Design review of the part shown in the three views and the two pictorial views. Dimensions are in mm from the part's minimum x, y and z. A direction names the side the tool comes from. Coordinates: 2 decimals unless noted, no trailing zeros. Loops run counter-clockwise (first coordinate to the right, second up) from the corner with the lowest first, then second, coordinate; pieces in that order, holes last. Notation, with made-up numbers: (9, -21) - (63, -21) arc R22 ccw to (63, 8) - close; hole circle Ø1 at (82.5, 82). An arc over 180 degrees is marked (long way). One line per item, written item: value. Start each with the question number.
1. Take a section at A-A, the plane z = 49. State the section outline as (x, y) points (1 decimal), and give its area (3 significant figures).
2. Take a section at B-B, the plane x = 25. State the section outline as (y, z) points (1 decimal), and give its area (3 significant figures).
3. To check wall thickness, follow line 1 (X direction, y = 6.1, z = 5.08) (1 decimal); line 2 (X direction, y = 5, z = 69) (1 decimal); line 3 (Y direction, x = 5.5, z = 97) (1 decimal). State the ranges of each line that lie inside material, in increasing order. Write a range as from..to.
4. For the marked faces 1, 2 and 3, list the 3-axis set-ups (+Z, -Z, +X, -X, +Y, -Y) from which the entire face can be reached by the end or side of a thin tool; tool diameter is ignored.
5. Take a section at C-C, the plane z = 5.08. State the section outline as (x, y) points (1 decimal).
6. Insertion check: pin 1 (6 mm diameter, centred on x = 10.5, z = 27.5, fed in from -Y) (1 decimal); pin 2 (4 mm diameter, centred on x = 14.64, z = 109.22, fed in from -Y) (1 decimal); pin 3 (5 mm diameter, centred on x = 43.5, z = 26, fed in from +Y) (1 decimal). Each pin has a flat end and moves straight along its axis. Give the tip position at first contact, or say it passes through.
7. Take a section at D-D, the plane z = 23.5. State the section outline as (x, y) points (1 decimal).
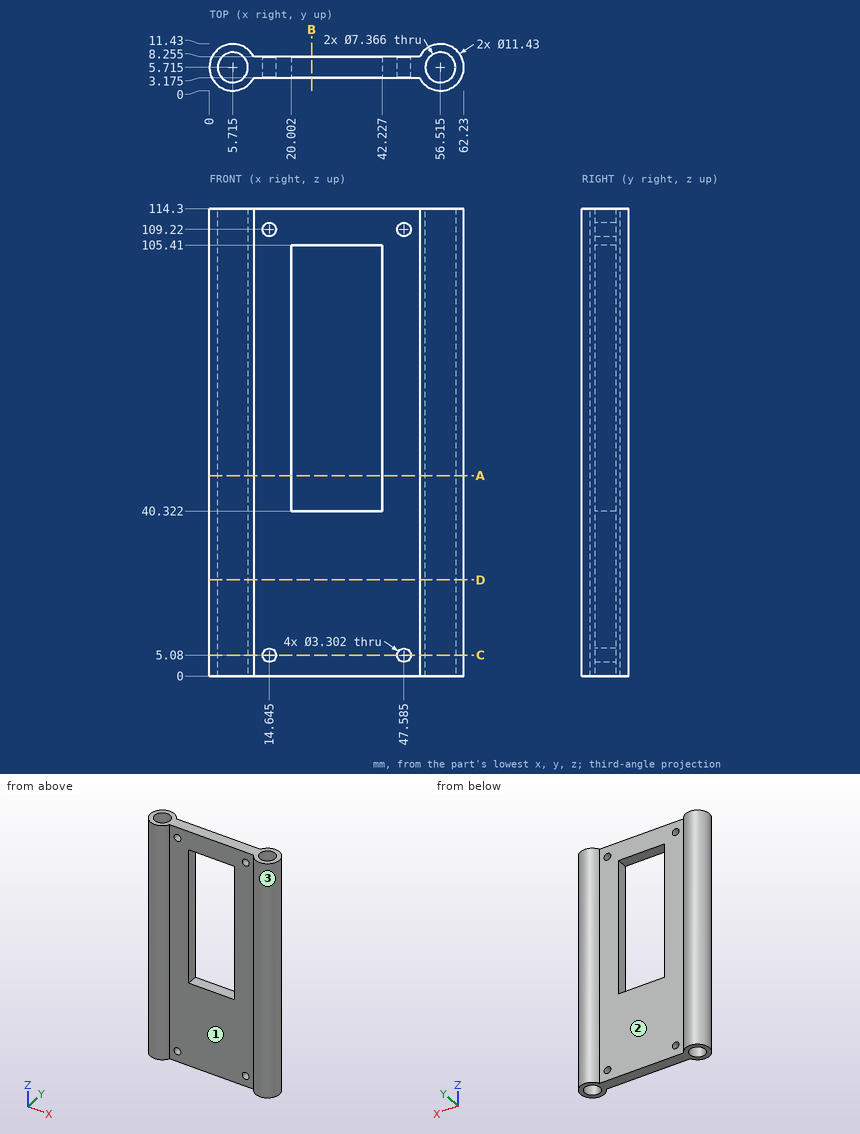
Solutions:
1. outline: (10.8, 3.2) - (20, 3.2) - (20, 8.3) - (10.8, 8.3) arc R5.7 ccw (long way) to start; (42.2, 3.2) - (51.4, 3.2) arc R5.7 ccw (long way) to (51.4, 8.3) - (42.2, 8.3) - close; hole circle Ø7.4 at (5.7, 5.7); hole circle Ø7.4 at (56.5, 5.7)
1. area: 209 mm2
2. outline: (3.2, 0) - (8.3, 0) - (8.3, 40.3) - (3.2, 40.3) - close; (3.2, 105.4) - (8.3, 105.4) - (8.3, 114.3) - (3.2, 114.3) - close
2. area: 250 mm2
3. line 1: 0..2.1, 9.4..13, 16.3..45.9, 49.2..52.9, 60.2..62.2
3. line 2: 0..2.1, 9.3..20, 42.2..52.9, 60.1..62.2
3. line 3: 0..2, 9.4..11.4
4. face 1: +Z, -Z, -Y
4. face 2: +Z, -Z, +Y
4. face 3: +Z, -Z
5. outline: (10.8, 3.2) - (13, 3.2) - (13, 8.3) - (10.8, 8.3) arc R5.7 ccw (long way) to start; (16.3, 3.2) - (45.9, 3.2) - (45.9, 8.3) - (16.3, 8.3) - close; (49.2, 3.2) - (51.4, 3.2) arc R5.7 ccw (long way) to (51.4, 8.3) - (49.2, 8.3) - close; hole circle Ø7.4 at (5.7, 5.7); hole circle Ø7.4 at (56.5, 5.7)
6. pin 1: y = 0.3
6. pin 2: y = 3.2
6. pin 3: y = 8.3
7. outline: (10.8, 3.2) - (51.4, 3.2) arc R5.7 ccw (long way) to (51.4, 8.3) - (10.8, 8.3) arc R5.7 ccw (long way) to start; hole circle Ø7.4 at (5.7, 5.7); hole circle Ø7.4 at (56.5, 5.7)
